Autodesk Inventor part; units mm, degrees
ref_plane "Arbeitsebene1" through (-6, 25, 0) normal (0.4226, 0, 0.9063) x (0.9063, 0, -0.4226)
ref_plane "YZ Plane" through (0, 0, 0) normal (1, 0, 0) x (0, 1, 0)
ref_plane "XZ Plane" through (0, 0, 0) normal (0, 1, 0) x (-1, 0, 0)
sketch "Skizze1" plane through (0, 0, 0) normal (0, 0, 1) x (1, 0, 0)
  line L0 (-6, -25) -> (6, -25)
  line L1 (6, -25) -> (6, 25)
  line L2 (6, 25) -> (-6, 25)
  line L3 (-6, 25) -> (-6, -25)
  line L4 (-6, -25) -> (6, 25) construction
  line L5 (6, -25) -> (-6, 25) construction
  line L6 (0, 20) -> (0, -20)
  point P0 (0, 0)
  point P1 (0, 0)
  dimension "d0" = 40
  dimension "d1" = 12
  dimension "d2" = 50
extrude "Extrusion1" add sketch "Skizze1" along normal blind 11
sketch "Skizze3" plane through (0, 0, 11) normal (0, 0, 1) x (1, 0, 0)
  line L0 (-6, -25) -> (6, -25)
  line L1 (6, -25) -> (6, 25)
  line L2 (6, 25) -> (-6, 25)
  line L3 (-6, 25) -> (-6, -25)
  point P0 (0, 0)
  point P1 (0, -20)
  point P2 (0, 20)
sketch "Skizze2" plane through (-6, -25, 0) normal (0, -1, 0) x (1, 0, 0)
  line L0 (0, 0) -> (12, 0)
  line L1 (12, 0) -> (12, 11)
  line L2 (0, 11) -> (12, 11)
  line L3 (0, 0) -> (0, 11)
  line L4 (0, 11) -> (12, 5.4043)
  point P0 (6, 0)
  dimension "d5" = 25
extrude "Extrusion2" cut sketch "Skizze2" against normal through all contours L2 L1 L4
hole "Bohrung1" at (0, 20, 11) at (0, -20, 11) direction (0, 0, -1) diameter 3 end through all counterbore diameter 4 counterbore depth 7
sketch "Skizze4" plane through (-6, -25, 11) normal (0.4226, 0, 0.9063) x (0.9063, 0, -0.4226)
  ellipse E0 centre (6.6203, 45) end of major axis (8.827, 45) minor radius 2
  ellipse E1 centre (6.6203, 5) end of major axis (8.827, 5) minor radius 2
  line L0 (0, 50) -> (13.2405, 50)
  line L1 (0, 50) -> (0, 0)
  line L2 (13.2405, 0) -> (0, 0)
  line L3 (13.2405, 50) -> (13.2405, 0)
  line L4 (6.6203, 12.5) -> (6.6203, 37.5)
  line L5 (0, 50) -> (0, 0)
  line L6 (0, 25) -> (13.2405, 25)
  line L7 (13.2405, 50) -> (13.2405, 0)
  point P0 (10.0866, 25)
  point P1 (6.6203, 25)
  dimension "d15" = 25
hole "Bohrung2" at (0, -12.5, 8.2022) at (0, 12.5, 8.2022) direction (-0.4226, 0, -0.9063) diameter 3 end through all
ref_plane "Arbeitsebene1" through (-6, 25, 0) normal (0.4226, 0, 0.9063) x (0.9063, 0, -0.4226)
sketch "Skizze5" plane through (-6, 25, 0) normal (0.4226, 0, 0.9063) x (0.9063, 0, -0.4226)
  circle A0 centre (1.9715, -37.5) radius 1.5
  circle A1 centre (1.9715, -12.5) radius 1.5
  ellipse E0 centre (1.9715, -5) end of major axis (4.1782, -5) minor radius 2
  ellipse E1 centre (1.9715, -45) end of major axis (4.1782, -45) minor radius 2
  line L0 (-4.6488, 0) -> (8.5917, 0)
  line L1 (-4.6488, 0) -> (-4.6488, -50)
  line L2 (8.5917, -50) -> (-4.6488, -50)
  line L3 (8.5917, 0) -> (8.5917, -50)
  point P0 (5.4378, -25)
hole "Bohrung3" at (-4.2132, 12.5, -0.8332) at (-4.2132, -12.5, -0.8332) direction (0.4226, 0, 0.9063) diameter 3 end through all counterbore diameter 4 counterbore depth 5
sketch "Skizze6" plane through (-6, -25, 0) normal (0, -1, 0) x (1, 0, 0)
  line L0 (12, 5.4043) -> (0, 11)
  line L1 (0, 0) -> (0, 11)
  line L2 (0, 0) -> (12, 0)
  line L3 (12, 0) -> (12, 5.4043)
  line L4 (12, 5.4043) -> (0, 9.772)
  point P0 (6, 0)
  dimension "d31" = 110
extrude "Extrusion3" cut sketch "Skizze6" against normal through all contours L4 L1 L0
properties part number "Mount_2"
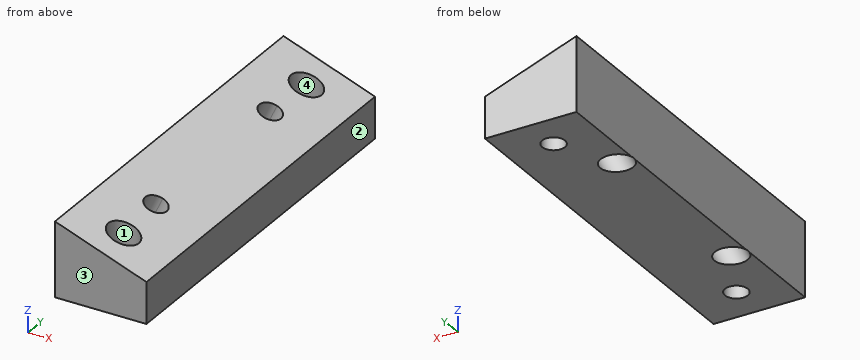
For this review, take the finished solid that the model builds, in its own axes (mm). Face numbers are marked on the shaded views. Round coordinates to 2 decimals unless told otherwise and drop trailing zeros. Loops run counter-clockwise (first coordinate to the right, second up) from the corner with the lowest first, then second, coordinate; pieces in that order, holes last.
Q1. Add section C-C on x = 4. Write out the cut boundary in (y, z).
Result sheet:
outline: (-25, 0) - (25, 0) - (25, 6.13) - (-25, 6.13) - close
Q2. Insertion check: pin 1 Ø3.5 at (x, y) = (0, -20) entering from +Z; pin 2 Ø5 at (x, y) = (1.5, -3) entering from +Z; pin 3 Ø4.5 at (x, y) = (-1, -19.5) entering from +Z. Each pin has a flat end and moves straight along its axis. Give the tip position at first contact, or say it passes through.
Result sheet:
pin 1: stops at z = 4
pin 2: stops at z = 7.95
pin 3: stops at z = 8.77
Q3. Add section A-A on y = -20. Write out the cut boundary in (x, z), plus the area to 3 significant figures.
Result sheet:
outline: (-6, 0) - (-1.5, 0) - (-1.5, 4) - (-2, 4) - (-2, 8.32) - (-6, 9.77) - close; (1.5, 0) - (6, 0) - (6, 5.4) - (2, 6.86) - (2, 4) - (1.5, 4) - close
area: 64.7 mm2
Q4. Add section B-B on y = -3. Write out the cut boundary in (x, z).
Result sheet:
outline: (-6, 0) - (6, 0) - (6, 5.4) - (-6, 9.77) - close
Q5. Mouldability with a two-part tool opening along Y and no side actions: class the marked faces 1, 2, 3 and 4 as +Y half, -Y half, draft (parallel to the pull), parting line (faces both ways), or undercut.
Result sheet:
face 1: undercut
face 2: draft
face 3: -Y half
face 4: undercut
Q6. To check wall thickness, follow line 1 along Y through (x, z) = (0, 3); line 2 along X through (y, z) = (-20, 1.5); line 3 along Y through (x, z) = (0, 7.05). State the ranges of each line that lie inside material, in increasing order.
Result sheet:
line 1: y = -25 to -21.5, -18.5 to 18.5, 21.5 to 25
line 2: x = -6 to -1.5, 1.5 to 6
line 3: y = -25 to -22, -18 to -13.92, -11.08 to 11.08, 13.92 to 18, 22 to 25
